Here's how the part is built. I have some questions about the finished solid (model axes, mm). Face numbers are marked on the shaded views. A direction names the side the tool comes from. Give positions to 0.01 mm unless a question says otherwise; leave off trailing zeros. Loops run counter-clockwise (first coordinate to the right, second up) from the corner with the lowest first, then second, coordinate; pieces in that order, holes last. Notation, with made-up numbers: (-29, 42.25) - (5, 42.25) arc R19 ccw to (5, 62.25) - close; hole circle Ø1 at (61.5, 87.25). An arc over 180 degrees is marked (long way). Use a Markdown table: item, result.
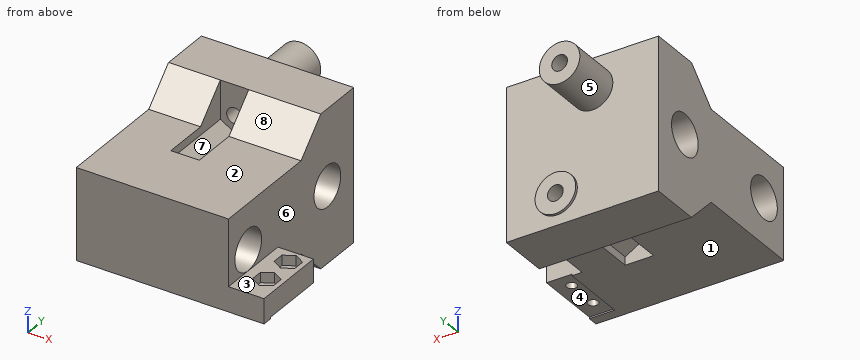
from build123d import *

# Parameters (mm, degrees)
SKETCH_1_W          = 30
SKETCH_1_H          = 30
EXTRUDE_1_DEPTH     = 38
SKETCH_3_R          = 4
EXTRUDE_3_DEPTH     = 0.5
SKETCH_7_R          = 4
EXTRUDE_4_DEPTH     = 10
SKETCH_6_R          = 4.05
CUT_EXTRUDE_3_DEPTH = 31
SKETCH_9_R          = 1.55
CUT_EXTRUDE_4_DEPTH = 21
CUT_EXTRUDE_6_DEPTH = 31
CUT_EXTRUDE_5_DEPTH = 15
SKETCH_12_W         = 4.9
SKETCH_12_H         = 15
EXTRUDE_5_DEPTH     = 7
SKETCH_13_W         = 5
SKETCH_13_H         = 13
CUT_EXTRUDE_7_DEPTH = 0.3
SKETCH_14_R         = 1
CUT_EXTRUDE_8_DEPTH = 24.7
CUT_EXTRUDE_9_DEPTH = 2


with BuildPart() as part:
    # 草图1 → 凸台-拉伸1 (new body)
    with BuildSketch(Plane(origin=(0, 0, 0), x_dir=(1, 0, 0), z_dir=(0, 1, 0))):
        with Locations((15, 15)):
            Rectangle(SKETCH_1_W, SKETCH_1_H)
    extrude(amount=EXTRUDE_1_DEPTH)

    # 草图3 → 凸台-拉伸3 (add)
    with BuildSketch(Plane(origin=(0, 38, -50), x_dir=(1, 0, 0), z_dir=(0, -1, 0))):
        with Locations((20, 26)):
            Circle(SKETCH_3_R)
    extrude(amount=-EXTRUDE_3_DEPTH)

    # 草图7 → 凸台-拉伸4 (add)
    with BuildSketch(Plane.XZ.offset(-38)):
        with Locations((13, -6)):
            Circle(SKETCH_7_R)
    extrude(amount=-EXTRUDE_4_DEPTH)

    # 草图6 → 切除-拉伸3 (cut, through all)
    with BuildSketch(Plane(origin=(30, 0, 0), x_dir=(0, 0, -1), z_dir=(1, 0, 0))):
        with Locations((15, 6)):
            Circle(SKETCH_6_R)
        with Locations((15, 30)):
            Circle(SKETCH_6_R)
    extrude(amount=-CUT_EXTRUDE_3_DEPTH, mode=Mode.SUBTRACT)

    # 草图9 → 切除-拉伸4 (cut, through all)
    with BuildSketch(Plane(origin=(0, 28, 0), x_dir=(1, 0, 0), z_dir=(0, 1, 0))):
        with Locations((13, 6)):
            Circle(SKETCH_9_R)
        with Locations((20, 24)):
            Circle(SKETCH_9_R)
    extrude(amount=CUT_EXTRUDE_4_DEPTH, mode=Mode.SUBTRACT)

    # 草图11 → 切除-拉伸6 (cut, through all)
    with BuildSketch(Plane(origin=(30, 0, 0), x_dir=(0, 0, -1), z_dir=(1, 0, 0))):
        Polygon((6, 0), (6, 22), (0, 28), (0, 0), align=None)
        Polygon((24, 0), (24, 22), (30, 28), (30, 0), align=None)
    extrude(amount=-CUT_EXTRUDE_6_DEPTH, mode=Mode.SUBTRACT)

    # 草图10 → 切除-拉伸5 (cut)
    with BuildSketch(Plane(origin=(0, 28, 0), x_dir=(1, 0, 0), z_dir=(0, 1, 0))):
        Polygon((15.8, 0), (15.8, 7.616580754), (13, 9.233161507), (10.2, 7.616580754), (10.2, 0), align=None)
        Polygon((20, 20.766838493), (22.8, 22.383419246), (22.8, 30), (17.2, 30), (17.2, 22.383419246), align=None)
    extrude(amount=-CUT_EXTRUDE_5_DEPTH, mode=Mode.SUBTRACT)

    # 草图12 → 凸台-拉伸5 (add)
    with BuildSketch(Plane(origin=(30, 0, 0), x_dir=(0, 0, -1), z_dir=(1, 0, 0))):
        with Locations((21.55, 7.5)):
            Rectangle(SKETCH_12_W, SKETCH_12_H)
    extrude(amount=EXTRUDE_5_DEPTH)

    # 草图13 → 切除-拉伸7 (cut)
    with BuildSketch(Plane(origin=(0, 0, -24), x_dir=(-1, 0, 0), z_dir=(0, 0, -1))):
        with Locations((-34.5, 8.5)):
            Rectangle(SKETCH_13_W, SKETCH_13_H)
    extrude(amount=-CUT_EXTRUDE_7_DEPTH, mode=Mode.SUBTRACT)

    # 草图14 → 切除-拉伸8 (cut, through all)
    with BuildSketch(Plane(origin=(0, 0, -23.7), x_dir=(-1, 0, 0), z_dir=(0, 0, -1))):
        with Locations((-34, 12)):
            Circle(SKETCH_14_R)
        with Locations((-34, 5.5)):
            Circle(SKETCH_14_R)
    extrude(amount=-CUT_EXTRUDE_8_DEPTH, mode=Mode.SUBTRACT)

    # 草图15 → 切除-拉伸9 (cut)
    with BuildSketch(Plane.XY.offset(-19.1)):
        Polygon((36.05, 10.816431948), (36.05, 13.183568052), (34, 14.367136104), (31.95, 13.183568052), (31.95, 10.816431948), (34, 9.632863896), align=None)
        Polygon((34, 3.132863896), (36.05, 4.316431948), (36.05, 6.683568052), (34, 7.867136104), (31.95, 6.683568052), (31.95, 4.316431948), align=None)
    extrude(amount=-CUT_EXTRUDE_9_DEPTH, mode=Mode.SUBTRACT)


solid = part.part
(1) Will these pins go through, and if not, where does the flat tip stop? pin 1 (3.5 mm diameter, centred on x = 34, y = 5, fed in from +Z); pin 2 (1 mm diameter, centred on x = 20.5, z = -22.5, fed in from +Y); pin 3 (8.5 mm diameter, centred on y = 23, z = -5, fed in from +X); pin 4 (4 mm diameter, centred on x = 23, y = 41, fed in from -Z).
A:
| item | result |
|---|---|
| pin 1 | z = -19.1 |
| pin 2 | y = 38.5 |
| pin 3 | x = 30 |
| pin 4 | through |
(2) Suppose I cut it at B-B on x = 3. Write out the boundary of the cut face in (y, z), plus the area to 3 significant figures.
A:
| item | result |
|---|---|
| outline | (0, -24) - (22, -24) - (28, -30) - (38, -30) - (38, 0) - (28, 0) - (22, -6) - (0, -6) - close; hole circle Ø8.1 at (6, -15); hole circle Ø8.1 at (30, -15) |
| area | 737 mm2 |
(3) Suppose I cut it at A-A on y = 12. Write out the boundary of the cut face in (x, z).
A:
| item | result |
|---|---|
| outline | (0, -24) - (32, -24) - (32, -23.7) - (33, -23.7) - (33, -21.1) - (31.95, -21.1) - (31.95, -19.1) - (30, -19.1) - (30, -6) - (0, -6) - close; (35, -23.7) - (37, -23.7) - (37, -19.1) - (36.05, -19.1) - (36.05, -21.1) - (35, -21.1) - close |
(4) On a 3-axis mill with a long thin cutter (end or side, diameter ignored), from which of +Z, -Z, +X, -X, +Y, -Y can I reach the whole of each face in a straight line? I mean the marked faces 1, 2, 3 and 4. Say none if no direction works.
A:
| item | result |
|---|---|
| face 1 | -Z, +X, -X, -Y |
| face 2 | +Z, +X, -X, -Y |
| face 3 | +Z, +X, +Y, -Y |
| face 4 | -Z, +X, +Y |
(5) If I drill on line 1 (Y direction, x = 16, z = -15); line 2 (Y direction, x = 34, z = -22.1); line 3 (X direction, y = 20, z = -7), over which ranges is the centre line in solid material (lowest first)?
A:
| item | result |
|---|---|
| line 1 | 0 to 1.95, 10.05 to 25.95, 34.05 to 38 |
| line 2 | 0 to 4.5, 6.5 to 11, 13 to 15 |
| line 3 | 0 to 10.2, 15.8 to 30 |
(6) We'd pull the mould along X, two halves only. Please class the marked faces 5, 6, 7 and 8: pulls with the +X half, pulls with the -X half, needs draft (parallel to the pull), parting line crosses it, or undercut.
A:
| item | result |
|---|---|
| face 5 | parting line crosses it |
| face 6 | pulls with the +X half |
| face 7 | undercut |
| face 8 | needs draft |
(7) Suppose I cut it at C-C on z = -15. Write out the boundary of the cut face in (x, y), plus the area to 3 significant figures.
A:
| item | result |
|---|---|
| outline | (0, 0) - (30, 0) - (30, 1.95) - (0, 1.95) - close; (0, 10.05) - (30, 10.05) - (30, 25.95) - (0, 25.95) - close; (0, 34.05) - (30, 34.05) - (30, 38) - (0, 38) - close |
| area | 654 mm2 |
(8) Suppose I cut it at D-D on x = 19. Write out the boundary of the cut face in (y, z), plus the area to 3 significant figures.
A:
| item | result |
|---|---|
| outline | (0, -24) - (13, -24) - (13, -21.34) - (28, -21.34) - (28, -22.82) - (38.5, -22.82) - (38.5, -20.13) - (38, -20.13) - (38, 0) - (28, 0) - (22, -6) - (0, -6) - close; (28, -30) - (38, -30) - (38, -27.87) - (38.5, -27.87) - (38.5, -25.18) - (28, -25.18) - close; hole circle Ø8.1 at (6, -15); hole circle Ø8.1 at (30, -15) |
| area | 658 mm2 |
